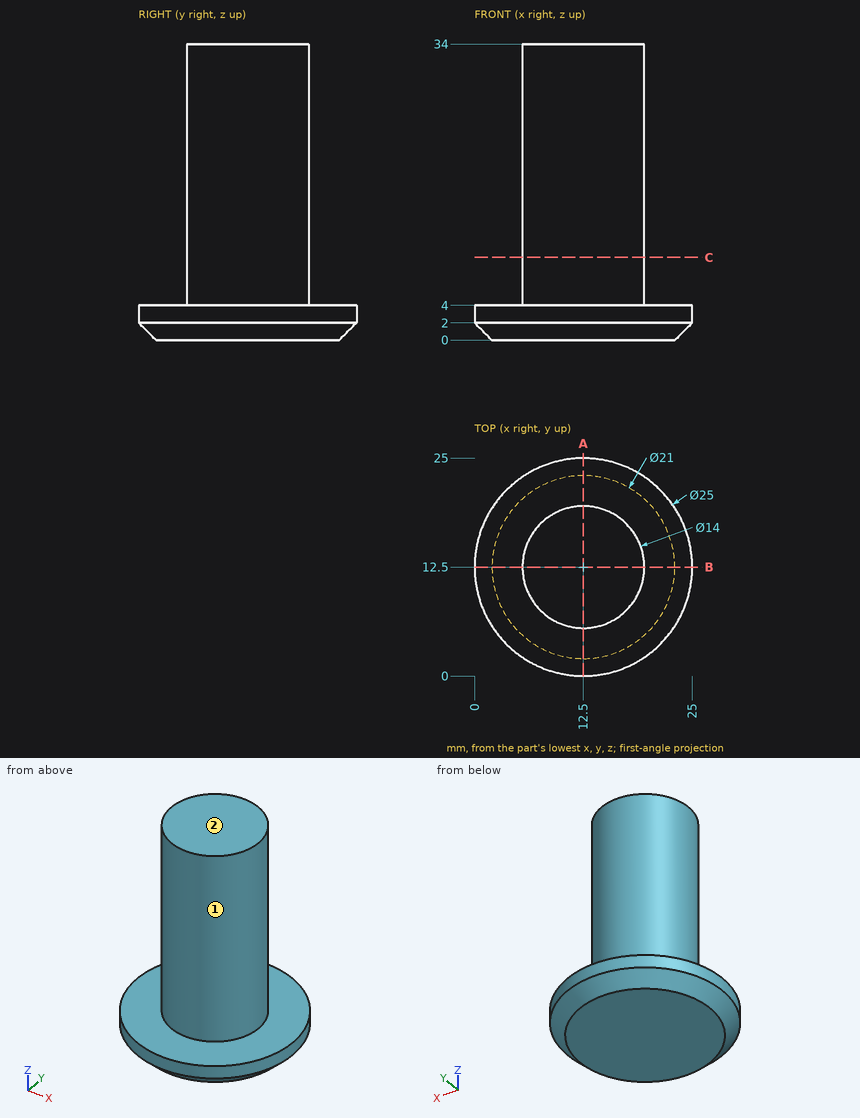
Input: dimensioned drawing with shaded views. Units: mm. Origin: part minimum x, y, z. A direction names the side the tool comes from. Give positions to 0.01 mm unless a question says otherwise; leave off trailing zeros. Write each loop counter-clockwise with the first axis right and the second up, starting at its lowest first coordinate (ties: lowest second). Pieces come first, ordered by that corner, then holes.
1. Line query: probe 1 along Z at (x, y) = (5.75, 17.75); probe 2 along X at (y, z) = (12.75, 30); probe 3 along Y at (x, z) = (7.75, 12). Output: solid intervals per line, ascending.
2. Pin query (flat end, axial travel): P1, Ø1, axis at y = 21.5, z = 25, coming from the -X side; P2, Ø8, axis at y = 12, z = 18, coming from the -X side; P3, Ø5, axis at x = 7, z = 25.5, coming from the -Y side; P4, Ø8, axis at y = 6, z = 24, coming from the -X side. Return the tip coordinate at first contact, or that it passes through.
3. Section query C-C, the plane z = 9.5. Return loops of the section in (x, y), then the cut area to 3 significant figures.
4. Reachability of the marked faces 1 and 2 from +Z, -Z, +X, -X, +Y, -Y: full face, straight path, thin tool, end or side. Return the list, or none.
5. Section query A-A, the plane x = 12.5. Return loops of the section in (y, z).
Computed:
1. probe 1: z = 0 to 4
1. probe 2: x = 5.5 to 19.5
1. probe 3: y = 7.36 to 17.64
2. P1: passes through
2. P2: stops at x = 5.5
2. P3: stops at y = 6.18
2. P4: stops at x = 5.96
3. outline: circle Ø14 at (12.5, 12.5)
3. area: 154 mm2
4. face 1: +Z
4. face 2: +Z, +X, -X, +Y, -Y
5. outline: (0, 2) - (2, 0) - (23, 0) - (25, 2) - (25, 4) - (19.5, 4) - (19.5, 34) - (5.5, 34) - (5.5, 4) - (0, 4) - close
